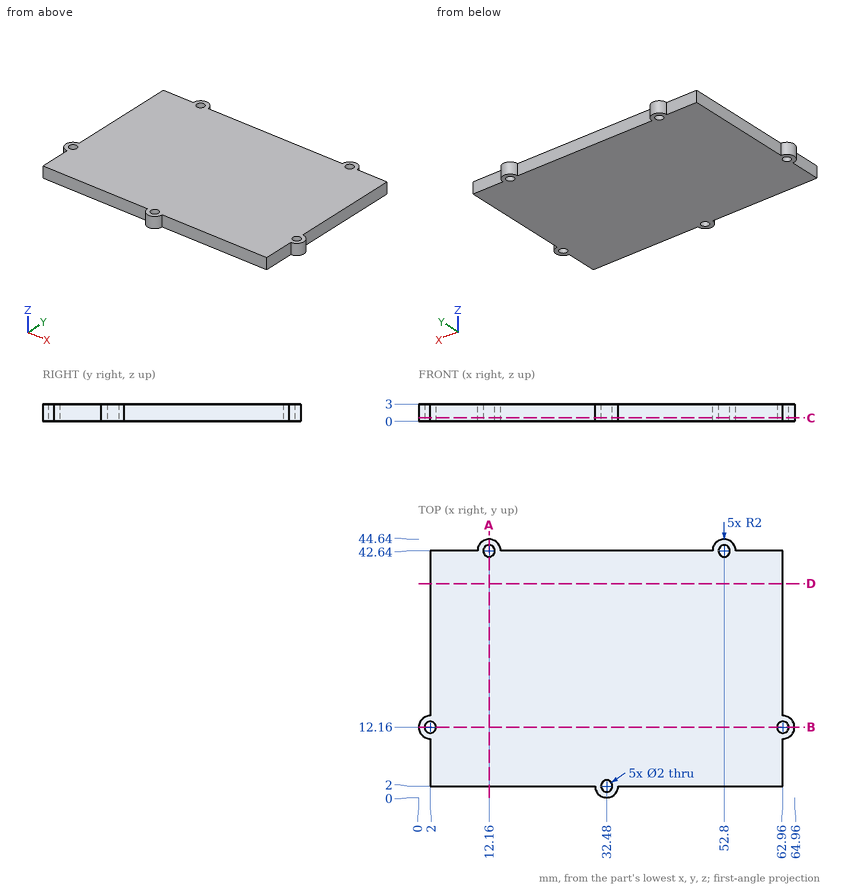
Here's the drawing with two shaded views (mm, measured from the low corner). I have some questions. Coordinates: 2 decimals unless noted, no trailing zeros. Loops run counter-clockwise (first coordinate to the right, second up) from the corner with the lowest first, then second, coordinate; pieces in that order, holes last. Notation, with made-up numbers: (11.25, -29.5) -> (39.25, -29.5) arc R8 ccw to (39.25, -18.5) -> close; hole circle Ø11 at (8, -10). An arc over 180 degrees is marked (long way). Put each result on its own line as item: value. Start each with the question number.
Q1. I want a section at D-D (y = 37). Write out the boundary of the cut face in (x, z).
Q2. I want a section at B-B (y = 12.16). Write out the boundary of the cut face in (x, z).
Q3. I want a section at C-C (z = 0.6). Write out the boundary of the cut face in (x, y), plus the area to 3 significant figures.
Q4. If I drill on line 1 (X direction, y = 11.5, z = 0.95); line 2 (Y direction, x = 12.16, z = 1.9); line 3 (Y direction, x = 32.48, z = 1.35), over which ranges is the centre line in solid material (lowest first)? Write a range as [from, to].
Q5. I want a section at A-A (x = 12.16). Write out the boundary of the cut face in (y, z).
Q6. I'm going to push flat-ended pins straight in: P1, Ø1, axis at y = 15.5, z = 1.5, coming from the -X side; P2, Ø2.5, axis at x = 52.8, y = 42.64, coming from the -Z side; P3, Ø0.9, axis at x = 36.5, z = 1, coming from the +Y side; P4, Ø1.2, axis at x = 12.16, y = 42.64, coming from the +Z side. Where does each tip first touch, or does it pass through?
Taken from the geometry:
1. outline: (2, 0) -> (62.96, 0) -> (62.96, 3) -> (2, 3) -> close
2. outline: (0, 0) -> (1, 0) -> (1, 3) -> (0, 3) -> close; (3, 0) -> (61.96, 0) -> (61.96, 3) -> (3, 3) -> close; (63.96, 0) -> (64.96, 0) -> (64.96, 3) -> (63.96, 3) -> close
3. outline: (2, 2) -> (30.48, 2) arc R2 ccw to (34.48, 2) -> (62.96, 2) -> (62.96, 10.16) arc R2 ccw to (62.96, 14.16) -> (62.96, 42.64) -> (54.8, 42.64) arc R2 ccw to (50.8, 42.64) -> (14.16, 42.64) arc R2 ccw to (10.16, 42.64) -> (2, 42.64) -> (2, 14.16) arc R2 ccw to (2, 10.16) -> close; hole circle Ø2 at (2, 12.16); hole circle Ø2 at (12.16, 42.64); hole circle Ø2 at (32.48, 2); hole circle Ø2 at (52.8, 42.64); hole circle Ø2 at (62.96, 12.16)
3. area: 2,490 mm2
4. line 1: x = [0.11, 1.25], [2.75, 62.21], [63.71, 64.85]
4. line 2: y = [2, 41.64], [43.64, 44.64]
4. line 3: y = [0, 1], [3, 42.64]
5. outline: (2, 0) -> (41.64, 0) -> (41.64, 3) -> (2, 3) -> close; (43.64, 0) -> (44.64, 0) -> (44.64, 3) -> (43.64, 3) -> close
6. P1: stops at x = 2
6. P2: stops at z = 0
6. P3: stops at y = 42.64
6. P4: passes through
